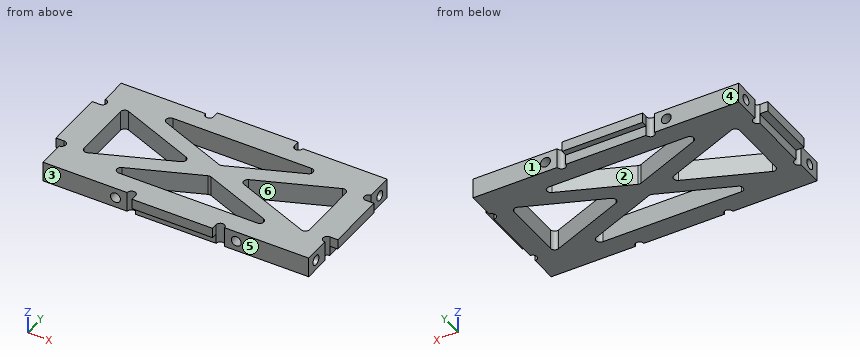
Autodesk Inventor part; units mm, degrees
ref_plane "YZ Plane" through (0, 0, 0) normal (1, 0, 0) x (0, 1, 0)
ref_plane "XZ Plane" through (0, 0, 0) normal (0, 1, 0) x (-1, 0, 0)
ref_plane "XY Plane" through (0, 0, 0) normal (0, 0, 1) x (1, 0, 0)
sketch "スケッチ1" plane through (0, 0, 0) normal (0, 0, 1) x (1, 0, 0)
  line L0 (-33, 9.6) -> (-33, 16.25)
  line L1 (-33, 16.25) -> (-20, 16.25)
  line L2 (20, 16.25) -> (33, 16.25)
  line L3 (33, 16.25) -> (33, 9.6)
  line L4 (0, 0) -> (0, 16.25) construction
  line L5 (0, 0) -> (35, 0) construction
  line L6 (33, 7.5) -> (35, 7.5)
  line L7 (35, 7.5) -> (35, -7.5)
  line L8 (35, -7.5) -> (33, -7.5)
  line L9 (-20, -16.25) -> (20, -16.25) construction
  line L10 (20, -16.25) -> (20, 16.25) construction
  line L11 (20, 16.25) -> (-20, 16.25) construction
  line L12 (-20, 16.25) -> (-20, -16.25) construction
  line L13 (-20, -16.25) -> (20, 16.25) construction
  line L14 (20, -16.25) -> (-20, 16.25) construction
  line L15 (-33, -16.25) -> (33, -16.25) construction
  line L16 (33, -16.25) -> (33, 16.25) construction
  line L17 (33, 16.25) -> (-33, 16.25) construction
  line L18 (-33, 16.25) -> (-33, -16.25) construction
  line L19 (-33, -16.25) -> (33, 16.25) construction
  line L20 (33, -16.25) -> (-33, 16.25) construction
  arc A0 (33, 9.6) -> (33, 7.5) centre (33, 8.55) ccw
  arc A1 (33, -7.5) -> (33, -9.6) centre (33, -8.55) ccw
  line L21 (33, -9.6) -> (33, -16.25)
  line L22 (33, -16.25) -> (20, -16.25)
  line L23 (20, -16.25) -> (12.1, -16.25)
  line L24 (-20, 16.25) -> (-12.1, 16.25)
  line L25 (-10, 16.25) -> (-10, 17.75)
  line L26 (-10, 17.75) -> (10, 17.75)
  line L27 (10, 17.75) -> (10, 16.25)
  line L28 (20, 16.25) -> (12.1, 16.25)
  arc A2 (-12.1, 16.25) -> (-10, 16.25) centre (-11.05, 16.25) ccw
  arc A3 (10, 16.25) -> (12.1, 16.25) centre (11.05, 16.25) ccw
  line L29 (-33, 7.5) -> (-35, 7.5)
  line L30 (-35, 7.5) -> (-35, -7.5)
  line L31 (-35, -7.5) -> (-33, -7.5)
  arc A4 (-33, 7.5) -> (-33, 9.6) centre (-33, 8.55) ccw
  arc A5 (-33, -9.6) -> (-33, -7.5) centre (-33, -8.55) ccw
  line L32 (-33, -9.6) -> (-33, -16.25)
  line L33 (-33, -16.25) -> (-20, -16.25)
  line L34 (-20, -16.25) -> (-12.1, -16.25)
  line L35 (-10, -16.25) -> (-10, -17.75)
  line L36 (-10, -17.75) -> (10, -17.75)
  line L37 (10, -17.75) -> (10, -16.25)
  arc A6 (-10, -16.25) -> (-12.1, -16.25) centre (-11.05, -16.25) ccw
  arc A7 (12.1, -16.25) -> (10, -16.25) centre (11.05, -16.25) ccw
  line L38 (-16.55, 19.1799) -> (-13.45, 19.1799) construction
  line L39 (-13.45, 19.1799) -> (-13.45, 12.4242) construction
  line L40 (-13.45, 12.4242) -> (-16.55, 12.4242) construction
  line L41 (-16.55, 12.4242) -> (-16.55, 19.1799) construction
  line L42 (-15, 19.1799) -> (-15, 12.4242) construction
  point P0 (0, 17.75)
  point P1 (0, 0)
  dimension "d0" = 1.05
  dimension "d1" = 32.5
  dimension "d2" = 66
  dimension "d3" = 40
  dimension "d23" = 2
  dimension "d30" = 1.5
  dimension "d34" = 8.75
  dimension "d53" = 20
  dimension "d54" = 3.1
  dimension "d55" = 5
  dimension "d85" = 32.5
extrude "押し出し1" add sketch "スケッチ1" along normal blind 5
sketch "スケッチ2" plane through (0, 0, 0) normal (0, 0, -1) x (-1, 0, 0)
  line L0 (33, 9.6) -> (33, 16.25)
  line L1 (-33, 16.25) -> (-33, 9.6)
  line L2 (-41.1427, 17.3125) -> (-33, 17.3125)
  line L3 (-33, 17.3125) -> (-33, -16.751)
  line L4 (-33, -16.751) -> (-41.1427, -16.751)
  line L5 (-41.1427, -16.751) -> (-41.1427, 17.3125)
  line L6 (33, 21.1805) -> (38.858, 21.1805)
  line L7 (38.858, 21.1805) -> (38.858, -13.6193)
  line L8 (38.858, -13.6193) -> (33, -13.6193)
  line L9 (33, -13.6193) -> (33, 21.1805)
  line L10 (-20, -16.25) -> (-12.1, -16.25)
  line L11 (-17.1371, 25.1848) -> (11.8342, 25.1848)
  line L12 (11.8342, 25.1848) -> (11.8342, 16.25)
  line L13 (11.8342, 16.25) -> (-17.1371, 16.25)
  line L14 (-17.1371, 16.25) -> (-17.1371, 25.1848)
  line L15 (-13.151, -21.5857) -> (17.7795, -21.5857)
  line L16 (17.7795, -21.5857) -> (17.7795, -16.25)
  line L17 (17.7795, -16.25) -> (-13.151, -16.25)
  line L18 (-13.151, -16.25) -> (-13.151, -21.5857)
  line L19 (-12.1, 16.25) -> (-33, 16.25)
  line L20 (-33, -16.25) -> (-12.1, -16.25)
  point P0 (0, 0)
extrude "押し出し2" cut sketch "スケッチ2" against normal blind 2.5
sketch "スケッチ3" plane through (12.1, 16.25, 0) normal (0, 1, 0) x (1, 0, 0)
  line L0 (-2.1, 0) -> (-2.1, -5)
  line L1 (-2.1, -5) -> (-22.1, -5) construction
  line L2 (-12.1, -5) -> (-12.1, 7.4607) construction
  line L3 (20.9, 0) -> (20.9, -5)
  point P0 (-12.1, 0)
  point P1 (2.9, -2.5)
  point P2 (-27.1, -2.5)
  point P3 (20.9, -2.5)
  dimension "d60" = 5
hole "穴1" at (15, 16.25, 2.5) at (-15, 16.25, 2.5) direction (0, -1, 0) diameter 2.459 depth 2.5
mirror "ミラー1" about plane through (0, 0, 0) normal (0, 1, 0) of "穴1"
sketch "スケッチ4" plane through (33, -16.25, 5) normal (1, 0, 0) x (0, 0, -1)
  line L0 (5, 16.25) -> (0, 16.25) construction
  line L1 (0, 23.75) -> (0, 8.75) construction
  line L2 (5, 6.65) -> (0, 6.65)
  line L3 (5, 0) -> (0, 0)
  point P0 (2.5, 3)
  point P1 (2.5, 29.5)
  point P2 (2.5, 6.65)
  dimension "d86" = 3
  dimension "d87" = 26.5
hole "穴2" at (33, -13.25, 2.5) at (33, 13.25, 2.5) direction (-1, 0, 0) diameter 2.459 depth 2.5
mirror "ミラー2" about plane through (0, 0, 0) normal (1, 0, 0) of "穴2"
sketch "スケッチ5" plane through (0, 0, 0) normal (0, 0, -1) x (-1, 0, 0)
  line L0 (10, 16.25) -> (-10, 16.25)
  line L1 (-33, 7.5) -> (-33, 9.6)
  line L2 (-28, -11.25) -> (28, -11.25) construction
  line L3 (28, -11.25) -> (28, 11.25) construction
  line L4 (28, 11.25) -> (-28, 11.25) construction
  line L5 (-28, 11.25) -> (-28, -11.25) construction
  line L6 (-28, -11.25) -> (28, 11.25) construction
  line L7 (28, -11.25) -> (-28, 11.25) construction
  line L8 (-28, 9.0946) -> (-28, -9.0946)
  line L9 (-28, -9.0946) -> (-5.3645, 0)
  line L10 (-5.3645, 0) -> (-28, 9.0946)
  line L11 (-22.6355, 11.25) -> (22.6355, 11.25)
  line L12 (22.6355, 11.25) -> (0, 2.1554)
  line L13 (0, 2.1554) -> (-22.6355, 11.25)
  line L14 (-22.6355, -11.25) -> (22.6355, -11.25)
  line L15 (22.6355, -11.25) -> (0, -2.1554)
  line L16 (0, -2.1554) -> (-22.6355, -11.25)
  line L17 (28, 9.0946) -> (28, -9.0946)
  line L18 (28, -9.0946) -> (5.3645, 0)
  line L19 (5.3645, 0) -> (28, 9.0946)
  point P0 (-12.1, 16.25)
  point P1 (-20, 16.25)
  point P2 (-33, 16.25)
  point P3 (0, 0)
  dimension "d76" = 5
  dimension "d77" = 5
  dimension "d78" = 4
  dimension "d79" = 4
  dimension "d80" = 4
  dimension "d81" = 4
extrude "押し出し3" cut sketch "スケッチ5" against normal blind 10
fillet "フィレット1" radius 1.05 12 edges at (28, 9.0946, 2.5) (28, -9.0946, 2.5) (22.6355, 11.25, 2.5) (5.3645, 0, 2.5) (0, -2.1554, 2.5) (0, 2.1554, 2.5) (-28, -9.0946, 2.5) (22.6355, -11.25, 2.5) (-28, 9.0946, 2.5) (-22.6355, 11.25, 2.5) (-22.6355, -11.25, 2.5) (-5.3645, 0, 2.5)
equation "\"d85\" = d1"
equation "\"d77\" = d76"
equation "\"d79\" = d78"
equation "\"d80\" = d79"
equation "\"d81\" = d78"
equation "\"d52\" = 5"
properties part number "胴体_メインフレーム_1_13" material "アセタール樹脂、黒"
Input: part model. Units: mm. Frame: model coordinates. Face numbers are marked on the shaded views. A direction names the side the tool comes from. Give positions to 0.01 mm unless a question says otherwise; leave off trailing zeros. Order: outer loops, then holes, each group sorted by start corner. A loop starts at its lowest first (then second) coordinate and runs counter-clockwise, first axis right, second up. Notation, with made-up numbers: M 30,40.25 L 73,40.25 A11 cw 73,46.25 Z; hole C -37.75,-18.5 d3. An arc over 180 degrees is marked long. Return JSON: item names as keys, results as strings.
Item 1: Pull-direction query (Y, two-part tool) for the marked faces 1, 2 and 3; classes: +Y half, -Y half, draft (parallel to the pull), parting line (faces both ways), or undercut.
Solutions:
{"face 1": "+Y half", "face 2": "undercut", "face 3": "-Y half"}
Item 2: Cut plane A-A (x = -25.5). Return loops of the section in (y, z), then the cut area to 3 significant figures.
Solutions:
{"outline": "M -16.25,0 L -8.09,0 L -8.09,5 L -16.25,5 Z; M 8.09,0 L 16.25,0 L 16.25,5 L 8.09,5 Z", "area": "81.6 mm^2"}
Item 3: Cut plane B-B (y = 6.5). Return loops of the section in (x, z).
Solutions:
{"outline": "M -35,2.5 L -33,2.5 L -33,0 L -28,0 L -28,5 L -35,5 Z; M -21.54,0 L -10.81,0 L -10.81,5 L -21.54,5 Z; M 10.81,0 L 21.54,0 L 21.54,5 L 10.81,5 Z; M 28,0 L 33,0 L 33,2.5 L 35,2.5 L 35,5 L 28,5 Z"}
Item 4: Cut plane C-C (x = 11.05). Return loops of the section in (y, z), then the cut area to 3 significant figures.
Solutions:
{"outline": "M -15.2,0 L -11.25,0 L -11.25,5 L -15.2,5 Z; M -6.6,0 L -2.28,0 L -2.28,5 L -6.6,5 Z; M 2.28,0 L 6.6,0 L 6.6,5 L 2.28,5 Z; M 11.25,0 L 15.2,0 L 15.2,5 L 11.25,5 Z", "area": "82.6 mm^2"}
Item 5: First-contact query: P1, Ø0.6, axis at x = 33.5, z = 3, coming from the +Y side; P2, Ø2.5, axis at y = 12.5, z = 1.5, coming from the +X side; P3, Ø2, axis at y = -13.25, z = 2.5, coming from the -X side. Flat tips, straight axial feed; report the tip coordinate or a pass-through.
Solutions:
{"P1": "y = 7.5", "P2": "x = 33", "P3": "x = -30.5"}
Item 6: Ray query, probe 1 along Y at (x, z) = (31.6, 2.5); probe 2 along X at (y, z) = (15, 2.5); probe 3 along X at (y, z) = (-5, 2.4). Return the intervals inside material, ascending.
Solutions:
{"probe 1": "-16.25 to -14.48, -12.02 to 12.02, 14.48 to 16.25", "probe 2": "-33 to -16.23, -13.77 to 13.77, 16.23 to 33", "probe 3": "-33 to -28, -17.81 to -7.08, 7.08 to 17.81, 28 to 33"}
Item 7: Access query for the marked faces 4, 5 and 6. Directions: +Z, -Z, +X, -X, +Y, -Y. A direction counts if a zero-diameter tool reaches every point of the face in a straight line with its end or side. Return the directions, or none.
Solutions:
{"face 4": "+Z, -Z, -X, +Y", "face 5": "+Z, -Z, +X, -Y", "face 6": "+Z, -Z"}
